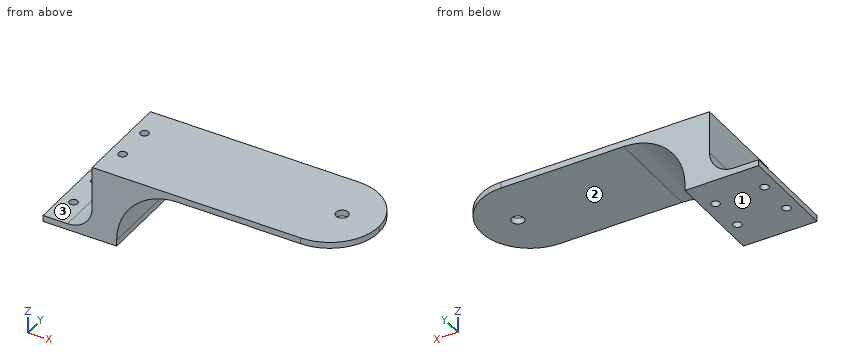
from build123d import *

# Parameters (mm, degrees)
BOSS_EXTRUDE1_DEPTH = 3.175
SKETCH2_W           = 12.7
SKETCH2_H           = 50.8
BOSS_EXTRUDE2_DEPTH = 31.75
FILLET1_R           = 12.7
BOSS_EXTRUDE3_DEPTH = 3.175
FILLET2_R           = 31.75
SKETCH4_R           = 2.15265
CUT_EXTRUDE1_DEPTH  = 38.1
FILLET3_R           = 25.4
CUT_EXTRUDE4_REACH  = 131.047
SKETCH7_R           = 3.175


with BuildPart() as part:
    # Sketch1 → Boss-Extrude1 (new body)
    with BuildSketch(Plane.XY.offset(15.875)):
        Polygon((-38.1, 25.4), (-38.1, -25.4), (-25.4, -25.4), (0, -25.4), (0, 25.4), align=None)
    extrude(amount=BOSS_EXTRUDE1_DEPTH)

    # Sketch2 → Boss-Extrude2 (add)
    with BuildSketch(Plane.XY.offset(50.8)):
        with Locations((-6.35, 0)):
            Rectangle(SKETCH2_W, SKETCH2_H)
    extrude(amount=-BOSS_EXTRUDE2_DEPTH)

    # Fillet1
    fillet1_edges = [part.edges().sort_by_distance(p)[0] for p in [
        (-12.7, 0, 19.05),
    ]]
    fillet(fillet1_edges, radius=FILLET1_R)

    # Sketch3 → Boss-Extrude3 (add)
    with BuildSketch(Plane.XY.offset(50.8)):
        Polygon((0, 25.4), (101.6, 25.4), (120.65, 25.4), (120.65, -25.4), (0, -25.4), (-12.7, -25.4), (-12.7, 25.4), align=None)
    extrude(amount=BOSS_EXTRUDE3_DEPTH)

    # Fillet2
    fillet2_edges = [part.edges().sort_by_distance(p)[0] for p in [
        (0, 0, 50.8),
    ]]
    fillet(fillet2_edges, radius=FILLET2_R)

    # Sketch4 → Cut-Extrude1 (cut)
    with BuildSketch(Plane.XY.offset(53.975)):
        with Locations((-6.35, 9.525)):
            Circle(SKETCH4_R)
        with Locations((-31.75, 9.525)):
            Circle(SKETCH4_R)
        with Locations((-6.35, -9.525)):
            Circle(SKETCH4_R)
        with Locations((-31.75, -9.525)):
            Circle(SKETCH4_R)
    extrude(amount=-CUT_EXTRUDE1_DEPTH, mode=Mode.SUBTRACT)

    # Fillet3
    fillet3_edges = [part.edges().sort_by_distance(p)[0] for p in [
        (120.65, -25.4, 52.3875),
        (120.65, 25.4, 52.3875),
    ]]
    fillet(fillet3_edges, radius=FILLET3_R - 0.0001)  # a hair under: the kernel refuses the full size

    # Sketch7 → Cut-Extrude4 (cut, up to next)
    with BuildSketch(Plane.XY.offset(53.975), mode=Mode.PRIVATE) as cut_extrude4_sk1:
        with Locations((101.6, 0)):
            Circle(SKETCH7_R)
    cut_extrude4_tool1 = extrude(cut_extrude4_sk1.sketch, amount=-CUT_EXTRUDE4_REACH, mode=Mode.PRIVATE) & part.part
    add(cut_extrude4_tool1.solids().sort_by_distance((101.6, 0, 53.975))[0], mode=Mode.SUBTRACT)


solid = part.part
Design review of the part built by this model. Coordinates are the model's own, in mm. Face numbers are marked on the shaded views. A direction names the side the tool comes from. Round coordinates to 2 decimals unless told otherwise and drop trailing zeros. Loops run counter-clockwise (first coordinate to the right, second up) from the corner with the lowest first, then second, coordinate; pieces in that order, holes last. Notation, with made-up numbers: (-10, 13.25) - (25, 13.25) arc R19 cw to (25, 45.25) - close; hole circle Ø3 at (66, -24). An arc over 180 degrees is marked (long way). One line per item, written item: value. Start each with the question number.
1) Consider section A-A on x = -31.75. Give the boundary of the cut face in (y, z) (3 decimals), then the cut area to 3 significant figures.
2) For the marked faces 1, 2 and 3, list the 3-axis set-ups (+Z, -Z, +X, -X, +Y, -Y) from which the entire face can be reached by the end or side of a thin tool; tool diameter is ignored.
3) Consider section C-C on x = 101.6. Give the boundary of the cut face in (y, z) (3 decimals).
4) To check wall thickness, follow L1, parallel to Y at x = -6, z = 27; L2, parallel to Y at x = -6.35, z = 31; L3, parallel to Z at x = 39, y = -3 (3 decimals). State the ranges of each line that lie inside material, in increasing order. Write a range as from..to.
5) Consider section D-D on x = -6.35. Give the boundary of the cut face in (y, z) (3 decimals).
6) Insertion check: pin 1 Ø2.5 at (y, z) = (11.5, 18) entering from +X; pin 2 Ø4 at (y, z) = (-17.5, 35) entering from -X; pin 3 Ø6.5 at (x, y) = (-29, 2) entering from +Z; pin 4 Ø5 at (x, y) = (-31.75, -9.525) entering from -Z (3 decimals). Each pin has a flat end and moves straight along its axis. Give the tip position at first contact, or say it passes through.
7) Consider section B-B on z = 39. Give the boundary of the cut face in (x, y) (3 decimals).
Reported:
1. outline: (-25.4, 15.875) - (-11.678, 15.875) - (-11.678, 19.05) - (-25.4, 19.05) - close; (-7.372, 15.875) - (7.372, 15.875) - (7.372, 19.05) - (-7.372, 19.05) - close; (11.678, 15.875) - (25.4, 15.875) - (25.4, 19.05) - (11.678, 19.05) - close
1. area: 134 mm^2
2. face 1: -Z, +X, -X, +Y, -Y
2. face 2: -Z, +X, +Y, -Y
2. face 3: +Z, -X, +Y, -Y
3. outline: (-24.593, 50.8) - (-3.175, 50.8) - (-3.175, 53.975) - (-24.593, 53.975) - close; (3.175, 50.8) - (24.593, 50.8) - (24.593, 53.975) - (3.175, 53.975) - close
4. L1: y = -25.4..-11.65, -7.4..7.4, 11.65..25.4
4. L2: y = -25.4..-11.68, -7.37..7.37, 11.68..25.4
4. L3: z = 50.8..53.975
5. outline: (-25.4, 15.875) - (-11.678, 15.875) - (-11.678, 53.975) - (-25.4, 53.975) - close; (-7.372, 15.875) - (7.372, 15.875) - (7.372, 53.975) - (-7.372, 53.975) - close; (11.678, 15.875) - (25.4, 15.875) - (25.4, 53.975) - (11.678, 53.975) - close
6. pin 1: stops at x = 0
6. pin 2: stops at x = -12.7
6. pin 3: stops at z = 19.05
6. pin 4: stops at z = 15.875
7. outline: (-12.7, -25.4) - (7.051, -25.4) - (7.051, 25.4) - (-12.7, 25.4) - close; hole circle Ø4.305 at (-6.35, -9.525); hole circle Ø4.305 at (-6.35, 9.525)
